Autodesk Inventor part; units mm, degrees
ref_plane "YZ Plane" through (0, 0, 0) normal (1, 0, 0) x (0, 1, 0)
ref_plane "XZ Plane" through (0, 0, 0) normal (0, 1, 0) x (-1, 0, 0)
ref_plane "XY Plane" through (0, 0, 0) normal (0, 0, 1) x (1, 0, 0)
sketch "Sketch1" plane through (0, 0, 0) normal (0, 0, 1) x (1, 0, 0)
  line L0 (0, 0) -> (90, 0)
  line L1 (90, 0) -> (90, 3)
  line L2 (90, 3) -> (0, 3)
  line L3 (0, 3) -> (0, 0)
  line L4 (0, 8) -> (90, 8)
  line L5 (90, 8) -> (90, 11)
  line L6 (90, 11) -> (0, 11)
  line L7 (0, 11) -> (0, 8)
  line L8 (0, 16) -> (90, 16)
  line L9 (90, 16) -> (90, 19)
  line L10 (90, 19) -> (0, 19)
  line L11 (0, 19) -> (0, 16)
  line L12 (0, 24) -> (90, 24)
  line L13 (90, 24) -> (90, 27)
  line L14 (90, 27) -> (0, 27)
  line L15 (0, 27) -> (0, 24)
  line L16 (0, 32) -> (90, 32)
  line L17 (90, 32) -> (90, 35)
  line L18 (90, 35) -> (0, 35)
  line L19 (0, 35) -> (0, 32)
  line L20 (0, 40) -> (90, 40)
  line L21 (90, 40) -> (90, 43)
  line L22 (90, 43) -> (0, 43)
  line L23 (0, 43) -> (0, 40)
  line L24 (0, 48) -> (90, 48)
  line L25 (90, 48) -> (90, 51)
  line L26 (90, 51) -> (0, 51)
  line L27 (0, 51) -> (0, 48)
  line L28 (0.0005, 56) -> (90.0005, 56)
  line L29 (90.0005, 56) -> (90.0005, 59)
  line L30 (90.0005, 59) -> (0.0005, 59)
  line L31 (0.0005, 59) -> (0.0005, 56)
  line L32 (0, 64) -> (90, 64)
  line L33 (90, 64) -> (90, 67)
  line L34 (90, 67) -> (0, 67)
  line L35 (0, 67) -> (0, 64)
  line L36 (0, 72) -> (90, 72)
  line L37 (90, 72) -> (90, 75)
  line L38 (90, 75) -> (0, 75)
  line L39 (0, 75) -> (0, 72)
  line L40 (0, 75) -> (90, 75)
  line L41 (90, 75) -> (90, 0)
  line L42 (90, 0) -> (0, 0)
  line L43 (0, 0) -> (0, 75)
  dimension "d0" = 3
  dimension "d1" = 90
  dimension "d2" = 3
  dimension "d3" = 90
  dimension "d4" = 3
  dimension "d5" = 90
  dimension "d6" = 3
  dimension "d7" = 90
  dimension "d8" = 3
  dimension "d9" = 90
  dimension "d10" = 3
  dimension "d11" = 90
  dimension "d12" = 3
  dimension "d13" = 90
  dimension "d14" = 3
  dimension "d15" = 90
  dimension "d16" = 3
  dimension "d17" = 90
  dimension "d18" = 3
  dimension "d19" = 90
  dimension "d20" = 5
  dimension "d21" = 5
  dimension "d22" = 5
  dimension "d23" = 5
  dimension "d24" = 5
  dimension "d25" = 5
  dimension "d26" = 5
  dimension "d27" = 5
  dimension "d28" = 5
extrude "Extrusion1" add sketch "Sketch1" against normal blind 65 contours L3 L2 L1 L0 | L7 L6 L5 L4 | L11 L10 L9 L8 | L15 L14 L13 L12 | L19 L18 L17 L16 | L23 L22 L21 L20 | L27 L26 L25 L24 | L31 L30 L29 L28 | L35 L34 L33 L32 | L39 L38 L37 L36
sketch "Sketch2" plane through (0, 0, 0) normal (0, 0, 1) x (1, 0, 0)
  point P0 (0, 0)
sketch "Sketch3" plane through (0, 0, 0) normal (0, 0, 1) x (1, 0, 0)
  line L0 (0, 72) -> (0, 75)
  line L1 (90, 0) -> (0, 0)
  line L2 (0, 0) -> (0, 75)
  line L3 (0, 75) -> (90, 75)
  line L4 (90, 75) -> (90, 0)
  line L5 (0, 75) -> (90, 75)
  line L6 (90, 75) -> (90, 95)
  line L7 (90, 95) -> (0, 95)
  line L8 (0, 95) -> (0, 75)
  line L9 (0, 0) -> (90, 0)
  line L10 (90, 0) -> (90, -20)
  line L11 (90, -20) -> (0, -20)
  line L12 (0, -20) -> (0, 0)
  point P0 (0, 0)
  dimension "d35" = 20
  dimension "d36" = 90
  dimension "d37" = 20
  dimension "d38" = 90
extrude "Extrusion2" add sketch "Sketch3" along normal blind 3 contours L0 L3 L4 L1 L2
sketch "Sketch4" plane through (0, 0, -65) normal (0, -1, 0) x (1, 0, 0)
  point P0 (0, 65)
sketch "Sketch5" plane through (0, 0, -65) normal (0, 0, -1) x (-1, 0, 0)
  line L0 (-90, 75) -> (0, 75)
  line L1 (-90, 75) -> (0, 75)
  line L2 (0, 75) -> (0, 0)
  line L3 (0, 0) -> (-90, 0)
  line L4 (-90, 0) -> (-90, 75)
extrude "Extrusion3" add sketch "Sketch5" along normal blind 3
properties part number "stack"
For this review, take the finished solid that the model builds, in its own axes (mm). Coordinates: 2 decimals unless noted, no trailing zeros. Answer as CSV lines item,"result". Start each with the question number.
1) Add section A-A (z = -39). Count the separate pieces of the cut face and the enclosed holes in it, then the cut area to 3 significant figures.
2) Draft analysis for pull direction Y (two halves, no side actions). For faces 1 (the flat face through (46, 67, -32)), 2 (the flat face through (44, 70, 0)), 3 (the flat face through (44, 38, 3)), 4 (the flat face through (44, 0, -32)), state which applies: +Y half, -Y half, draft (parallel to the pull), parting line (faces both ways), or undercut.
3) To check wall thickness, follow line 1 along Z through (x, y) = (13, 51.5). State the ranges of the line that lie inside material, in increasing order. Write a range as [from, to].
Result:
1,separate pieces,"10"
1,enclosed holes,"0"
1,area,"2,700 mm^2"
2,face 1,"undercut"
2,face 2,"undercut"
2,face 3,"draft"
2,face 4,"-Y half"
3,line 1,"[-68, -65], [0, 3]"
